```python
from build123d import *

# Parameters (mm, degrees)
F1_DEPTH       = 40
F2_W           = 100
F2_H           = 200
F3_DEPTH       = 100
F4_R           = 5
F5_T           = -2.5
F6_R           = 3
F7_DEPTH       = 25
F8_R           = 8
F9_DEPTH       = 25
F10_R          = 5.5
F11_DEPTH      = 25
F12_R          = 3
F12_R_2        = 1.25
F13_DEPTH      = 10
F14_R          = 3
F15_DEPTH      = 150
F17_START      = -41.94633
F16_W          = 15
F16_H          = 6
F17_DEPTH      = 208.05367
F18_R          = 1.5
F19_DEPTH      = 12.5
F20_R          = 6
F21_DEPTH      = 0.01
F21_DEPTH_BACK = 10
F22_R          = 3
F23_DEPTH      = 12.5
F24_R          = 2
F26_DEPTH      = 150


with BuildPart() as f1:
    # F0 (on Top) → F1 (new body)
    with BuildSketch(Plane.XY):
        with BuildLine():
            Line((-90, 83.2380757938), (-90, -50))
            Line((-90, -50), (90, -50))
            Line((90, -50), (90, 83.2380757938))
            ThreePointArc((90, 83.2380757938), (45.7737973711, 95.7737973711), (0, 100))
            ThreePointArc((0, 100), (-45.7737973711, 95.7737973711), (-90, 83.2380757938))
        make_face()
    extrude(amount=F1_DEPTH)

    # F2 (on Top) → F3 (cut)
    with BuildSketch(Plane.XY):
        with Locations((-120, -100)):
            Rectangle(F2_W, F2_H)
        with Locations((120, -100)):
            Rectangle(F2_W, F2_H)
    extrude(amount=F3_DEPTH, mode=Mode.SUBTRACT)

    # F4
    f4_edges = [f1.edges().sort_by_distance(p)[0] for p in [
        (-90, 83.238076, 20),
        (90, 83.238076, 20),
        (90, 0, 20),
        (70, 0, 20),
        (-90, 0, 20),
        (-70, 0, 20),
    ]]
    fillet(f4_edges, radius=F4_R)

    # F5
    f5_openings = [f1.faces().sort_by_distance(p)[0] for p in [
        (0, 26.262097, 40),
        (0, -50, 20),
    ]]
    offset(amount=F5_T, openings=f5_openings)

    # F6 (on Top) → F7 (cut)
    with BuildSketch(Plane.XY):
        with Locations((-55.8614357137, -24.1385642863)):
            Circle(F6_R)
        with Locations((55.8614357137, -24.1385642863)):
            Circle(F6_R)
    extrude(amount=F7_DEPTH, mode=Mode.SUBTRACT)

    # F8 (on Top) → F9 (join)
    with BuildSketch(Plane.XY):
        with Locations((-81, 77)):
            Circle(F8_R)
        with Locations((81, 77)):
            Circle(F8_R)
    extrude(amount=F9_DEPTH)

    # F10 (on Top) → F11 (cut)
    with BuildSketch(Plane.XY):
        with Locations((-81, 77)):
            Circle(F10_R)
        with Locations((81, 77)):
            Circle(F10_R)
    extrude(amount=F11_DEPTH, mode=Mode.SUBTRACT)

    # F12 (on Top) → F13 (join)
    with BuildSketch(Plane.XY):
        with Locations((-55, 15)):
            Circle(F12_R)
        with Locations((-55, 15)):
            Circle(F12_R_2, mode=Mode.SUBTRACT)
        with Locations((-39.8, 65.8)):
            Circle(F12_R)
        with Locations((-39.8, 65.8)):
            Circle(F12_R_2, mode=Mode.SUBTRACT)
        with Locations((-11.9, 65.8)):
            Circle(F12_R)
        with Locations((-11.9, 65.8)):
            Circle(F12_R_2, mode=Mode.SUBTRACT)
        with Locations((-6.8, 13.7)):
            Circle(F12_R)
        with Locations((-6.8, 13.7)):
            Circle(F12_R_2, mode=Mode.SUBTRACT)
    extrude(amount=F13_DEPTH)

    # F14 (on Front) → F15 (cut, symmetric)
    with BuildSketch(Plane.XZ):
        with Locations((47, 14)):
            Circle(F14_R)
        with Locations((-47, 14)):
            Circle(F14_R)
    extrude(amount=F15_DEPTH, both=True, mode=Mode.SUBTRACT)

    # F16 (on Front) → F17 (cut)
    with BuildSketch(Plane.XZ.offset(F17_START)):
        with Locations((0, 5.5)):
            Rectangle(F16_W, F16_H)
    extrude(amount=-F17_DEPTH, mode=Mode.SUBTRACT)

    # F18 (on Top) → F19 (cut, symmetric)
    with BuildSketch(Plane.XY):
        with Locations((-3, 95)):
            Circle(F18_R)
        with Locations((3, 95)):
            Circle(F18_R)
    extrude(amount=F19_DEPTH, both=True, mode=Mode.SUBTRACT)

    # F20 (on Top) → F21 (join, two sides)
    with BuildSketch(Plane.XY) as f21_sk:
        with Locations((-35, 90)):
            Circle(F20_R)
        with Locations((35, 90)):
            Circle(F20_R)
    extrude(amount=-F21_DEPTH)
    extrude(f21_sk.sketch, amount=F21_DEPTH_BACK)

    # F22 (on face) → F23 (cut, symmetric)
    with BuildSketch(Plane(origin=(0, 0, 0), x_dir=(1, 0, 0), z_dir=(0, 0, -1))):
        with Locations((-35, -90)):
            Circle(F22_R)
        with Locations((35, -90)):
            Circle(F22_R)
    extrude(amount=F23_DEPTH, both=True, mode=Mode.SUBTRACT)

    # F24
    f24_edges = [f1.edges().sort_by_distance(p)[0] for p in [
        (-87.5, 72.33631, 13.75),
        (-78.687247, 84.658405, 13.75),
        (-32.339812, 95.378048, 6.25),
        (-39.085326, 94.394328, 6.25),
        (39.085326, 94.394328, 6.25),
        (32.339812, 95.378048, 6.25),
        (78.687247, 84.658405, 13.75),
        (87.5, 72.33631, 13.75),
    ]]
    fillet(f24_edges, radius=F24_R)

    # F25 (on Right) → F26 (cut, symmetric)
    with BuildSketch(Plane.YZ):
        with BuildLine():
            Line((40, 20), (40, 30))
            ThreePointArc((40, 30), (35, 25), (40, 20))
        make_face()
        with BuildLine():
            ThreePointArc((65, 25), (63.5355339059, 28.5355339059), (60, 30))
            Line((60, 30), (60, 20))
            ThreePointArc((60, 20), (63.5355339059, 21.4644660941), (65, 25))
        make_face()
        with BuildLine():
            Line((60, 30), (40, 30))
            ThreePointArc((40, 30), (43.5355339059, 28.5355339059), (45, 25))
            ThreePointArc((45, 25), (43.5355339059, 21.4644660941), (40, 20))
            Line((40, 20), (60, 20))
            ThreePointArc((60, 20), (55, 25), (60, 30))
        make_face()
        with BuildLine():
            ThreePointArc((45, 25), (43.5355339059, 28.5355339059), (40, 30))
            Line((40, 30), (40, 20))
            ThreePointArc((40, 20), (43.5355339059, 21.4644660941), (45, 25))
        make_face()
        with BuildLine():
            Line((60, 20), (60, 30))
            ThreePointArc((60, 30), (55, 25), (60, 20))
        make_face()
    extrude(amount=F26_DEPTH, both=True, mode=Mode.SUBTRACT)


solid = f1.part
```
Verification items for the finished model (mm, model axes). A direction names the side the tool comes from. Coordinates: 2 decimals unless noted, no trailing zeros. Order: outer loops, then holes, each group sorted by start corner. A loop starts at its lowest first (then second) coordinate and runs counter-clockwise, first axis right, second up. Notation, with made-up numbers: (0, 30.5) - (16, 30.5) arc R16 cw to (16, 53.5) - close; hole circle Ø11 at (-18.5, 16.25). An arc over 180 degrees is marked (long way). Return JSON: item names as keys, results as strings.
(1) Section check D-D, the plane x = -26. Record the cut outline in (y, z).
Filled sheet:
{"outline": "(-50, 0) - (98.64, 0) - (98.64, 40) - (96.13, 40) - (96.13, 2.5) - (-50, 2.5) - close"}
(2) Section check A-A, the plane y = 43. Record the cut outline in (x, z), and give its area (4 significant figures).
Filled sheet:
{"outline": "(-90, 0) - (90, 0) - (90, 20) - (87.5, 20) - (87.5, 2.5) - (-87.5, 2.5) - (-87.5, 20) - (-90, 20) - close; (-90, 30) - (-87.5, 30) - (-87.5, 40) - (-90, 40) - close; (87.5, 30) - (90, 30) - (90, 40) - (87.5, 40) - close", "area": "587.5 mm^2"}
(3) Section check C-C, the plane z = 22.5. Give the number of separate pieces and of enclosed holes in the cut face, and give its area (3 significant figures).
Filled sheet:
{"separate pieces": "3", "enclosed holes": "2", "area": "1,230 mm^2"}
(4) Mould release check, pull along X, two halves, no side actions. Record for faces 1 (the flat face through (-7, 98, 40)), 2 (the cylindrical face through (-5.19, 16.23, 6.2)), 3 (the cylindrical face through (89, 2, 20)): pulls with the +X half, pulls with the -X half, needs draft (parallel to the pull), parting line crosses it, or undercut.
Filled sheet:
{"face 1": "needs draft", "face 2": "undercut", "face 3": "pulls with the +X half"}
(5) Access from +Z, -Z, +X, -X, +Y, -Y to the whole of each face (thin tool, end or side, straight path). Record for faces 4 (the flat face through (-80, 0, 20)), 5 (the cylindrical face through (-34.3, 84.04, 6.2)), 6 (the cylindrical face through (89.08, 82.67, 20.28)), 7 (the flat face through (-37, 87, 10)).
Filled sheet:
{"face 4": "+Z, -Z, -X, -Y", "face 5": "+Z", "face 6": "+Z, -Z, +X, +Y", "face 7": "+Z, -Y"}
(6) Go/stop test with flat-tipped pins: pin 1 (5 mm diameter, centred on x = -82.5, z = 27.5, fed in from +Y); pin 2 (1 mm diameter, centred on x = 53, z = 29, fed in from -Y); pin 3 (1 mm diameter, centred on x = -72, z = 25, fed in from +Y). Record where each tip stops, or that it passes through.
Filled sheet:
{"pin 1": "stops at y = 86.85", "pin 2": "stops at y = 91.65", "pin 3": "stops at y = 89.56"}
(7) Thickness scan on line 1 along X through (y, z) = (65.5, 34); line 2 along Y through (x, z) = (81, 5.5); line 3 along Y through (x, z) = (-39.8, 8). Record the ranges inside material, lowest first.
Filled sheet:
{"line 1": "x = -90 to -87.5, 87.5 to 90", "line 2": "y = 0 to 2.5, 69 to 71.5, 82.5 to 86.51", "line 3": "y = 62.8 to 64.55, 67.05 to 68.8, 86.4 to 96.81"}
